from build123d import *

# Parameters (mm, degrees)
SKETCH1_W                 = 38.1
SKETCH1_H                 = 38.1
BOSS_EXTRUDE1_DEPTH       = 5.8
SKETCH2_R                 = 8
CUT_EXTRUDE1_DEPTH        = 12.7
SKETCH4_R                 = 0.79375
CUT_EXTRUDE3_DEPTH        = 55.19280395
SKETCH6_W                 = 12.7
SKETCH6_H                 = 38.1
BOSS_EXTRUDE2_DEPTH       = 5.8
M3X0_5_TAPPED_HOLE1_D     = 2.5
M3X0_5_TAPPED_HOLE1_DEPTH = 7.5
M3X0_5_TAPPED_HOLE1_TIP   = 0.751075774
SKETCH9_R                 = 0.79375
CUT_EXTRUDE4_DEPTH        = 64.764331722
FILLET1_R                 = 6.35


with BuildPart() as part:
    # Sketch1 → Boss-Extrude1 (new body)
    with BuildSketch(Plane.XY):
        with Locations((-19.05, 19.05)):
            Rectangle(SKETCH1_W, SKETCH1_H)
    extrude(amount=BOSS_EXTRUDE1_DEPTH)

    # Sketch2 → Cut-Extrude1 (cut)
    with BuildSketch(Plane.XY.offset(5.8)):
        with Locations((-19.05, 19.05)):
            Circle(SKETCH2_R)
    extrude(amount=-CUT_EXTRUDE1_DEPTH, mode=Mode.SUBTRACT)

    # Sketch4 → Cut-Extrude3 (cut, through all)
    with BuildSketch(Plane.XY.offset(5.8)):
        with Locations((-34.925, 19.05)):
            Circle(SKETCH4_R)
        with Locations((-19.05, 34.925)):
            Circle(SKETCH4_R)
        with Locations((-3.175, 19.05)):
            Circle(SKETCH4_R)
        with Locations((-19.05, 3.175)):
            Circle(SKETCH4_R)
    extrude(amount=-CUT_EXTRUDE3_DEPTH, mode=Mode.SUBTRACT)

    # Sketch6 → Boss-Extrude2 (add, through all)
    with BuildSketch(Plane.XY.offset(5.8)):
        with Locations((6.35, 19.05)):
            Rectangle(SKETCH6_W, SKETCH6_H)
        with Locations((-44.45, 19.05)):
            Rectangle(SKETCH6_W, SKETCH6_H)
    extrude(amount=-BOSS_EXTRUDE2_DEPTH)

    # M3x0.5 Tapped Hole1
    with Locations(Plane.XY.offset(5.8)):
        with Locations((-44.45, 31.75), (6.35, 31.75), (6.35, 6.35), (-44.45, 6.35)):
            Hole(M3X0_5_TAPPED_HOLE1_D / 2, depth=M3X0_5_TAPPED_HOLE1_DEPTH)
            with Locations((0, 0, -(M3X0_5_TAPPED_HOLE1_DEPTH + M3X0_5_TAPPED_HOLE1_TIP / 2))):  # 118° drill point
                Cone(0, M3X0_5_TAPPED_HOLE1_D / 2, M3X0_5_TAPPED_HOLE1_TIP, mode=Mode.SUBTRACT)

    # Sketch9 → Cut-Extrude4 (cut, through all)
    with BuildSketch(Plane.XY.offset(5.8)):
        with Locations((-44.45, 19.05)):
            Circle(SKETCH9_R)
        with Locations((6.35, 19.05)):
            Circle(SKETCH9_R)
    extrude(amount=-CUT_EXTRUDE4_DEPTH, mode=Mode.SUBTRACT)

    # Fillet1
    fillet1_edges = [part.edges().sort_by_distance(p)[0] for p in [
        (12.7, 38.1, 2.9),
        (12.7, 0, 2.9),
        (-50.8, 0, 2.9),
        (-50.8, 38.1, 2.9),
    ]]
    fillet(fillet1_edges, radius=FILLET1_R)


solid = part.part
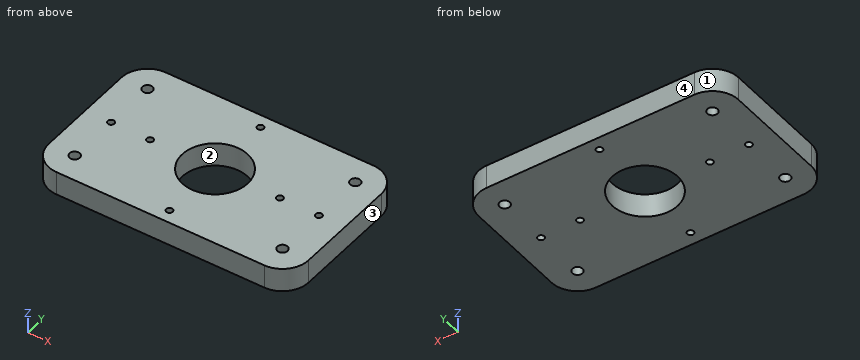
Geometry check sheet. Reference: the model listing, model coordinates, mm. Face numbers are marked on the shaded views. Give positions to 0.01 mm unless a question says otherwise; leave off trailing zeros. Loops run counter-clockwise (first coordinate to the right, second up) from the corner with the lowest first, then second, coordinate; pieces in that order, holes last. Notation, with made-up numbers: (84, 71) -> (117, 71) arc R22 ccw to (117, 94) -> close; hole circle Ø8 at (18, -19.75). An arc over 180 degrees is marked (long way). Answer in a Markdown table with one row per item. Add a question column.
1) Cross-section at B-B on x = -19.05. Record the boundary of the cut face in (y, z).
2) Material ranges on probe 1 along Y at (x, z) = (-44.5, 2.35); probe 2 along X at (y, z) = (6.5, 3.9); probe 3 along X at (y, z) = (31, 0.5), recorded low to high. Write a range as from..to.
3) Draft check along X on the marked faces 1, 2, 3 and 4. Enter one of: pulls with the +X half, pulls with the -X half, needs draft (parallel to the pull), parting line crosses it, or undercut.
4) Cross-section at C-C on z = 2.2. State how many separate pieces and enclosed holes the cut face has, and give its area (3 significant figures).
5) Gauge pin test, flat end, axial feed: P1, Ø1.5, axis at x = -44.45, y = 6.35, coming from the -Z side. Record the tip position at first contact, or that the pin passes through.
6) Cross-section at D-D on y = 7. Record the boundary of the cut face in (x, z).
7) Cross-section at A-A on y = 19.05. Record the boundary of the cut face in (x, z), and give its area (3 significant figures).
Outcome:
| question | item | result |
|---|---|---|
| 1 | outline | (0, 0) -> (2.38, 0) -> (2.38, 5.8) -> (0, 5.8) -> close; (3.97, 0) -> (11.05, 0) -> (11.05, 5.8) -> (3.97, 5.8) -> close; (27.05, 0) -> (34.13, 0) -> (34.13, 5.8) -> (27.05, 5.8) -> close; (35.72, 0) -> (38.1, 0) -> (38.1, 5.8) -> (35.72, 5.8) -> close |
| 2 | probe 1 | y = 0..5.1, 7.6..18.26, 19.84..30.5, 33..38.1 |
| 2 | probe 2 | x = -50.8..-45.69, -43.21..5.11, 7.59..12.7 |
| 2 | probe 3 | x = -50.8..-45.45, -43.45..5.35, 7.35..12.7 |
| 3 | face 1 | pulls with the -X half |
| 3 | face 2 | undercut |
| 3 | face 3 | pulls with the +X half |
| 3 | face 4 | needs draft |
| 4 | separate pieces | 1 |
| 4 | enclosed holes | 11 |
| 4 | area | 2,150 mm^2 |
| 5 | P1 | passes through |
| 6 | outline | (-50.8, 0) -> (-45.52, 0) -> (-45.52, 5.8) -> (-50.8, 5.8) -> close; (-43.38, 0) -> (5.28, 0) -> (5.28, 5.8) -> (-43.38, 5.8) -> close; (7.42, 0) -> (12.7, 0) -> (12.7, 5.8) -> (7.42, 5.8) -> close |
| 7 | outline | (-50.8, 0) -> (-45.24, 0) -> (-45.24, 5.8) -> (-50.8, 5.8) -> close; (-43.66, 0) -> (-35.72, 0) -> (-35.72, 5.8) -> (-43.66, 5.8) -> close; (-34.13, 0) -> (-27.05, 0) -> (-27.05, 5.8) -> (-34.13, 5.8) -> close; (-11.05, 0) -> (-3.97, 0) -> (-3.97, 5.8) -> (-11.05, 5.8) -> close; (-2.38, 0) -> (5.56, 0) -> (5.56, 5.8) -> (-2.38, 5.8) -> close; (7.14, 0) -> (12.7, 0) -> (12.7, 5.8) -> (7.14, 5.8) -> close |
| 7 | area | 239 mm^2 |
